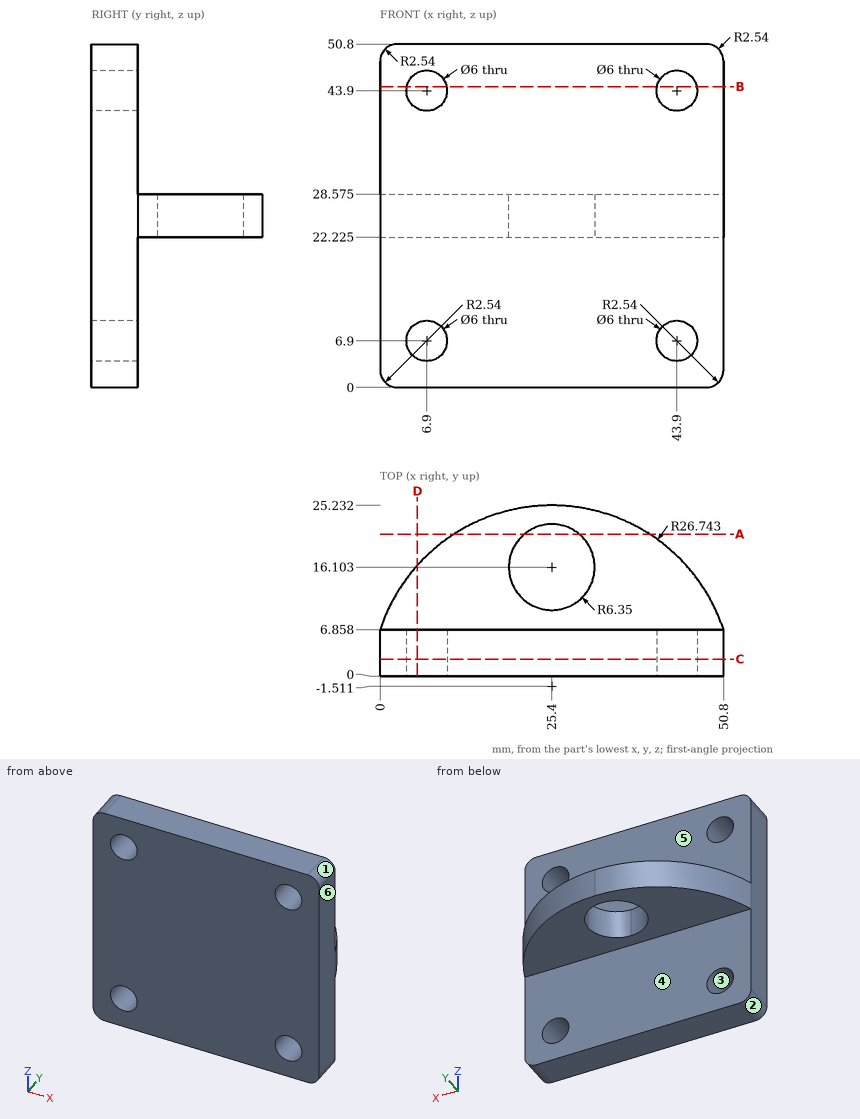
The drawing under review shows one solid part. Ordinate dimensions are in mm from its lowest x, y, z. A direction names the side the tool comes from. Coordinates: 2 decimals unless noted, no trailing zeros. Order: outer loops, then holes, each group sorted by start corner. A loop starts at its lowest first (then second) coordinate and runs counter-clockwise, first axis right, second up. Notation, with made-up numbers: (-32, 49.5) -> (19, 49.5) arc R35 cw to (19, 88.5) -> close; hole circle Ø5 at (20.5, 42). An arc over 180 degrees is marked (long way). Answer in a Markdown table with one row per item. Add a question column.
Item 1: We need section A-A on y = 21. Write out the cut boundary in (x, z) (1 decimal).
Item 2: Mouldability with a two-part tool opening along X and no side actions: class the marked faces 1, 2 and 3 as +X half, -X half, draft (parallel to the pull), parting line (faces both ways), or undercut.
Item 3: To check wall thickness, follow probe 1 along Z at (x, y) = (45.5, 2.75); probe 2 along Z at (x, y) = (6, 6.25); probe 3 along Z at (x, y) = (12, 13.75) (1 decimal). State the ranges of each line that lie inside material, in increasing order.
Item 4: We need section D-D on x = 5.5. Write out the cut boundary in (y, z) (1 decimal).
Item 5: Clearance check with flat-ended pins moving along their axes: pin 1 (1.5 mm diameter, centred on x = 10, y = 8, fed in from +Z) (3 decimals); pin 2 (6 mm diameter, centred on x = 29, y = 15.5, fed in from -Z) (3 decimals); pin 3 (8 mm diameter, centred on y = 15, z = 28, fed in from +X). State where each tip first meets the part, or that it passes through.
Item 6: We need section C-C on y = 2.5. Write out the cut boundary in (x, z), plus the area to 3 significant figures.
Item 7: Machinability: for the marked faces 4, 5 and 6, which of the approach directions +Z, -Z, +X, -X, +Y, -Y give a long, thin tool a straight path to every point of the face, cutting with its end or side? Answer none if there is none.
Item 8: We need section B-B on z = 44.5. Write out the cut boundary in (x, y), plus the area to 3 significant figures.
Final values:
| question | item | result |
|---|---|---|
| 1 | outline | (11, 22.2) -> (21.4, 22.2) -> (21.4, 28.6) -> (11, 28.6) -> close; (29.4, 22.2) -> (39.8, 22.2) -> (39.8, 28.6) -> (29.4, 28.6) -> close |
| 2 | face 1 | +X half |
| 2 | face 2 | -X half |
| 2 | face 3 | undercut |
| 3 | probe 1 | z = 0 to 4.36, 9.44 to 41.36, 46.44 to 50.8 |
| 3 | probe 2 | z = 0 to 4.04, 9.76 to 41.04, 46.76 to 50.8 |
| 3 | probe 3 | z = 22.2 to 28.6 |
| 4 | outline | (0, 0) -> (6.9, 0) -> (6.9, 4.2) -> (0, 4.2) -> close; (0, 9.6) -> (6.9, 9.6) -> (6.9, 22.2) -> (16.4, 22.2) -> (16.4, 28.6) -> (6.9, 28.6) -> (6.9, 41.2) -> (0, 41.2) -> close; (0, 46.6) -> (6.9, 46.6) -> (6.9, 50.8) -> (0, 50.8) -> close |
| 5 | pin 1 | stops at z = 28.575 |
| 5 | pin 2 | stops at z = 22.225 |
| 5 | pin 3 | stops at x = 49.04 |
| 6 | outline | (0, 2.54) arc R2.54 ccw to (2.54, 0) -> (48.26, 0) arc R2.54 ccw to (50.8, 2.54) -> (50.8, 48.26) arc R2.54 ccw to (48.26, 50.8) -> (2.54, 50.8) arc R2.54 ccw to (0, 48.26) -> close; hole circle Ø6 at (6.9, 6.9); hole circle Ø6 at (6.9, 43.9); hole circle Ø6 at (43.9, 6.9); hole circle Ø6 at (43.9, 43.9) |
| 6 | area | 2,460 mm2 |
| 7 | face 4 | -Z, +X, -X, +Y |
| 7 | face 5 | +Z, +X, -X, +Y |
| 7 | face 6 | +Z, -Z, +X, +Y, -Y |
| 8 | outline | (0, 0) -> (3.96, 0) -> (3.96, 6.86) -> (0, 6.86) -> close; (9.84, 0) -> (40.96, 0) -> (40.96, 6.86) -> (9.84, 6.86) -> close; (46.84, 0) -> (50.8, 0) -> (50.8, 6.86) -> (46.84, 6.86) -> close |
| 8 | area | 268 mm2 |
